```python
from build123d import *

# Parameters (mm, degrees)
SKETCH1_R           = 3.25
SKETCH1_R_2         = 5.25
SKETCH1_R_3         = 2.5
BOSS_EXTRUDE1_DEPTH = 10


with BuildPart() as part:
    # Sketch1 → Boss-Extrude1 (new body)
    with BuildSketch(Plane.XY):
        with BuildLine():
            Line((-42.222222222, -7.777777778), (-42.222222222, 42.222222222))
            Line((-42.222222222, 42.222222222), (-22.222222222, 42.222222222))
            Line((-22.222222222, 42.222222222), (-22.222222222, 32.222222222))
            Line((-22.222222222, 32.222222222), (-15.033488385, 32.222222222))
            ThreePointArc((-15.033488385, 32.222222222), (-2.53685568, 17.900528045), (15.60242755, 12.222222222))
            Line((15.60242755, 12.222222222), (52.777777778, 12.222222222))
            Line((52.777777778, 12.222222222), (52.777777778, -7.777777778))
            Line((52.777777778, -7.777777778), (32.777777778, -7.777777778))
            Line((32.777777778, -7.777777778), (32.777777778, -1.759068459))
            ThreePointArc((32.777777778, -1.759068459), (30.956018506, 0.70137381), (27.928044759, 1.152990889))
            Line((27.928044759, 1.152990889), (-18.776515477, 1.152990889))
            ThreePointArc((-18.776515477, 1.152990889), (-21.428517019, -0.376541989), (-22.222222222, -3.333333333))
            Line((-22.222222222, -3.333333333), (-22.222222222, -7.777777778))
            Line((-22.222222222, -7.777777778), (-42.222222222, -7.777777778))
        make_face()
        with Locations((-32.777777778, 34.166666667)):
            Circle(SKETCH1_R, mode=Mode.SUBTRACT)
        with Locations((-32.777777778, 4.166666667)):
            Circle(SKETCH1_R_2, mode=Mode.SUBTRACT)
        with Locations((-15.033488385, 17.900528045)):
            Circle(SKETCH1_R_3, mode=Mode.SUBTRACT)
        with Locations((42.5, 4.166666667)):
            Circle(SKETCH1_R_2, mode=Mode.SUBTRACT)
    extrude(amount=BOSS_EXTRUDE1_DEPTH)


solid = part.part
```
Read the model definition and answer for the solid it produces. Units are mm, in the model's axes. A direction names the side the tool comes from. Give positions to 0.01 mm unless a question says otherwise; leave off trailing zeros. Write each loop counter-clockwise with the first axis right and the second up, starting at its lowest first coordinate (ties: lowest second). Pieces come first, ordered by that corner, then holes. Notation, with made-up numbers: M 31,84.25 L 46,84.25 A22 ccw 46,112.25 Z; hole C 36.5,73 d3. An arc over 180 degrees is marked long. Put each result on its own line as item: value. Start each with the question number.
1. The part is cut by section A-A, the plane x = 42.5. Give the vertices of the cut face in (y, z).
2. Consider line 1 along X through (y, z) = (4, 9.25); line 2 along X through (y, z) = (0, 6.5); line 3 along X through (y, z) = (6, 6.5). Determine where each line is inside the solid, lowest interval first.
3. Each of these flat-tipped pins is pushed along its axis until it touches: pin 1 Ø1.5 at (x, y) = (-26.5, 12.5) entering from -Z; pin 2 Ø2 at (x, z) = (-17, 7.5) entering from +Y. Where does it stop, or does it pass through?
4. The part is cut by section D-D, the plane y = 28.5. Give the vertices of the cut face in (x, z), and give its area (3 significant figures).
5. The part is cut by section B-B, the plane y = 6. Give the vertices of the cut face in (x, z), and give its area (3 significant figures).
6. For a pull along X with two mould halves and no side action, classify faces 1 (the cylindrical face through (-31.031, 36.907, 4.93)), 2 (the flat face through (-42.222, 17, 5)), 3 (the cylindrical face through (-2.762, 18.049, 4.93)) as released by +X, released by -X, zero draft, split by the parting line, or undercut.
7. Which of the six approach directions +Z, -Z, +X, -X, +Y, -Y give full straight-line access (tool end or side, diameter ignored) to faces 4 (the flat face through (-22.222, 37, 5)), 5 (the cylindrical face through (-17.53, 18.01, 4.93)), 6 (the flat face through (-22.222, -6, 5))?
8. The part is cut by section C-C, the plane z = 5.5. Give the vertices of the cut face in (x, y).
Final values:
1. outline: M -7.78,0 L -1.08,0 L -1.08,10 L -7.78,10 Z; M 9.42,0 L 12.22,0 L 12.22,10 L 9.42,10 Z
2. line 1: x = -42.22 to -38.03, -27.53 to 37.25, 47.75 to 52.78
2. line 2: x = -42.22 to -35.97, -29.58 to -21.1, 31.82 to 39.31, 45.69 to 52.78
2. line 3: x = -42.22 to -37.7, -27.86 to 37.58, 47.42 to 52.78
3. pin 1: stops at z = 0
3. pin 2: stops at y = 32.22
4. outline: M -42.22,0 L -12.98,0 L -12.98,10 L -42.22,10 Z
4. area: 292 mm²
5. outline: M -42.22,0 L -37.7,0 L -37.7,10 L -42.22,10 Z; M -27.86,0 L 37.58,0 L 37.58,10 L -27.86,10 Z; M 47.42,0 L 52.78,0 L 52.78,10 L 47.42,10 Z
5. area: 753 mm²
6. face 1: undercut
6. face 2: released by -X
6. face 3: released by +X
7. face 4: +Z, -Z, +X, +Y
7. face 5: +Z, -Z
7. face 6: +Z, -Z, -Y
8. outline: M -42.22,-7.78 L -22.22,-7.78 L -22.22,-3.33 A4 cw -18.78,1.15 L 27.93,1.15 A4 cw 32.78,-1.76 L 32.78,-7.78 L 52.78,-7.78 L 52.78,12.22 L 15.6,12.22 A35 cw -15.03,32.22 L -22.22,32.22 L -22.22,42.22 L -42.22,42.22 Z; hole C -32.78,4.17 d10.5; hole C -32.78,34.17 d6.5; hole C -15.03,17.9 d5; hole C 42.5,4.17 d10.5
